Geometry: final body of the model. Coordinates: model frame, mm. Give positions to 0.01 mm unless a question says otherwise; leave off trailing zeros. Write each loop counter-clockwise with the first axis right and the second up, starting at its lowest first coordinate (ties: lowest second). Pieces come first, ordered by that corner, then holes.
Q1. Section A-A (x = 13.5). Return the cut outline in (y, z).
Q2. Pin query (flat end, axial travel): pin 1 Ø3 at (x, z) = (12, -3.5) entering from +Y; pin 2 Ø4 at (x, y) = (26, 2.5) entering from +Z; pin 3 Ø8 at (x, z) = (23.5, 6) entering from -Y. Return the tip coordinate at first contact, or that it passes through.
Q3. Line query: line 1 (Z direction, x = 37, y = 2.25); line 2 (Z direction, x = 20, y = -1.5); line 3 (Y direction, x = 10, z = -4.25). Output: solid intervals per line, ascending.
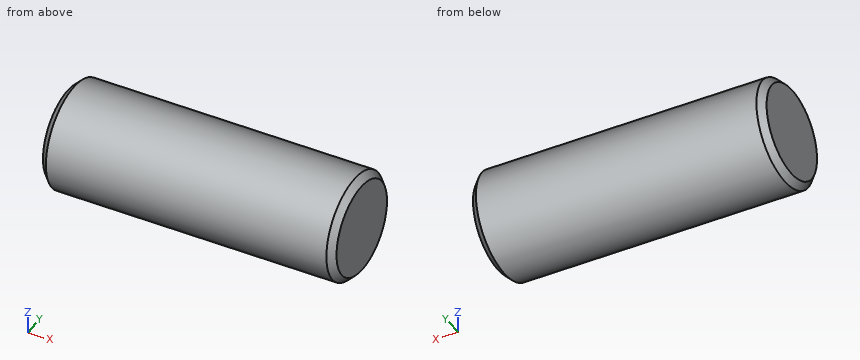
Autodesk Inventor part; units mm, degrees
ref_plane "YZ Plane" through (0, 0, 0) normal (1, 0, 0) x (0, 1, 0)
ref_plane "XZ Plane" through (0, 0, 0) normal (0, 1, 0) x (-1, 0, 0)
ref_plane "XY Plane" through (0, 0, 0) normal (0, 0, 1) x (1, 0, 0)
sketch "Эскиз1" plane through (0, 0, 0) normal (0, 0, 1) x (1, 0, 0)
  line L0 (0, 0) -> (0, 8)
  line L1 (0, 8) -> (45, 8)
  line L2 (45, 8) -> (45, 0)
  line L3 (0, 0) -> (45, 0)
  dimension "d0" = 45
  dimension "d1" = 16
revolve "Вращение1" add sketch "Эскиз1" angle 360 about axis through (0, 0, 0) along (1, 0, 0)
thread "Резьба1"
chamfer "Фаска1" distance 1 angle 45 1 edges at (45, -8, 0)
thread "Резьба2"
chamfer "Фаска2" distance 1 angle 45 1 edges at (0, -8, 0)
properties part number "Шпилька"
Computed:
1. outline: circle Ø16 at (0, 0)
2. pin 1: stops at y = 7.75
2. pin 2: stops at z = 7.98
2. pin 3: stops at y = -7.75
3. line 1: z = -7.68 to 7.68
3. line 2: z = -7.86 to 7.86
3. line 3: y = -6.78 to 6.78
